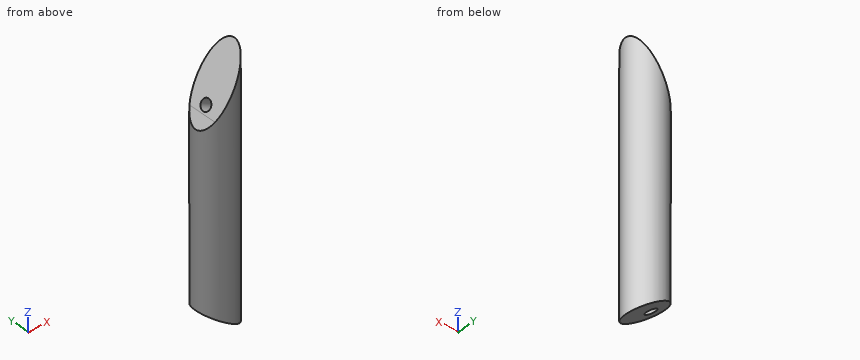
```python
from build123d import *

# Parameters (mm, degrees)
SKETCH1_R                 = 7.5
BOSS_EXTRUDE1_DEPTH       = 100
CUT_EXTRUDE1_DEPTH        = 8.5
CUT_EXTRUDE1_DEPTH_BACK   = 8.5
M5X0_8_TAPPED_HOLE2_D     = 4.2
M5X0_8_TAPPED_HOLE2_DEPTH = 10
M5X0_8_TAPPED_HOLE2_TIP   = 1.2618073
M5X0_8_TAPPED_HOLE3_D     = 4.2
M5X0_8_TAPPED_HOLE3_DEPTH = 7
M5X0_8_TAPPED_HOLE3_TIP   = 1.2618073


with BuildPart() as part:
    # Sketch1 → Boss-Extrude1 (new body)
    with BuildSketch(Plane.XY):
        Circle(SKETCH1_R)
    extrude(amount=BOSS_EXTRUDE1_DEPTH)

    # Sketch5 → Cut-Extrude1 (cut, two sides)
    with BuildSketch(Plane(origin=(0, 0, 0), x_dir=(1, 0, 0), z_dir=(0, 1, 0))) as cut_extrude1_sk:
        Polygon((7.5, 0), (-7.5, -8.660254038), (-7.5, 0), align=None)
        Polygon((7.5, -100), (-4.922116598, -78.484262915), (-7.5, -74.019237886), (-7.5, -100), align=None)
    extrude(amount=CUT_EXTRUDE1_DEPTH, mode=Mode.SUBTRACT)
    extrude(cut_extrude1_sk.sketch, amount=-CUT_EXTRUDE1_DEPTH_BACK, mode=Mode.SUBTRACT)

    # M5x0.8 Tapped Hole2
    with Locations(Plane(origin=(1.875, 0, 3.247595264), x_dir=(-0.866025404, 0, 0.5), z_dir=(-0.5, 0, -0.866025404))):
        with Locations((4.825317547, 0)):
            Hole(M5X0_8_TAPPED_HOLE2_D / 2, depth=M5X0_8_TAPPED_HOLE2_DEPTH)
            with Locations((0, 0, -(M5X0_8_TAPPED_HOLE2_DEPTH + M5X0_8_TAPPED_HOLE2_TIP / 2))):  # 118° drill point
                Cone(0, M5X0_8_TAPPED_HOLE2_D / 2, M5X0_8_TAPPED_HOLE2_TIP, mode=Mode.SUBTRACT)

    # M5x0.8 Tapped Hole3
    with Locations(Plane(origin=(-37.676270189, 0, 21.752404736), x_dir=(0.5, 0, 0.866025404), z_dir=(-0.866025404, 0, 0.5))):
        with Locations((68.352540378, 0)):
            Hole(M5X0_8_TAPPED_HOLE3_D / 2, depth=M5X0_8_TAPPED_HOLE3_DEPTH)
            with Locations((0, 0, -(M5X0_8_TAPPED_HOLE3_DEPTH + M5X0_8_TAPPED_HOLE3_TIP / 2))):  # 118° drill point
                Cone(0, M5X0_8_TAPPED_HOLE3_D / 2, M5X0_8_TAPPED_HOLE3_TIP, mode=Mode.SUBTRACT)


solid = part.part
```
Geometry check sheet. Reference: the model listing, model coordinates, mm. Coordinates: 2 decimals unless noted, no trailing zeros. Write each loop counter-clockwise with the first axis right and the second up, starting at its lowest first coordinate (ties: lowest second). Pieces come first, ordered by that corner, then holes. Notation, with made-up numbers: M 81,82 L 96,82 A32 cw 96,108 Z; hole C -8.75,-30.5 d11. An arc over 180 degrees is marked long. Use one line per item in the form item = value. Start each with the question number.
1) Go/stop test with flat-tipped pins: pin 1 Ø4 at (y, z) = (5, 52.5) entering from -X; pin 2 Ø6 at (y, z) = (-1.5, 79.5) entering from -X; pin 3 Ø1.5 at (x, y) = (2, -1.5) entering from +Z. Record where each tip stops, or that it passes through.
2) Thickness scan on probe 1 along Z at (x, y) = (2, -0.75); probe 2 along Y at (x, z) = (0.25, 23.5); probe 3 along X at (y, z) = (1.25, 19). Record the ranges inside material, lowest first. Write a range as from..to.
3) Section check D-D on x = 6.25. Enter the section's corners in (y, z).
4) Section check B-B on x = 2.5. State how many separate pieces and enclosed holes the cut face has, and give its area (3 significant figures).
5) Section check A-A on y = -4.5. Enter the section's corners in (x, z).
6) Section check C-C on z = 24.5. Enter the section's corners in (x, y).
Responses:
q1.pin_1 = -6.87
q1.pin_2 = -6.07
q1.pin_3 = 91.77
q2.probe_1 = 3.18..9.19, 15.27..76, 80.04..90.47
q2.probe_2 = -7.5..7.5
q2.probe_3 = -7.4..7.4
q3.outline = M -4.15,0.72 L 4.15,0.72 L 4.15,97.83 L -4.15,97.83 Z
q4.separate_pieces = 1
q4.enclosed_holes = 2
q4.area = 1,220 mm2
q5.outline = M -6,7.79 L 6,0.87 L 6,97.4 L -6,76.62 Z
q6.outline = C 0,0 d15
